Verification items for the finished model (mm, model axes). A direction names the side the tool comes from. Coordinates: 2 decimals unless noted, no trailing zeros. Order: outer loops, then holes, each group sorted by start corner. A loop starts at its lowest first (then second) coordinate and runs counter-clockwise, first axis right, second up.
Q1. Depth check by flat-ended pin: P1, Ø2, axis at x = 69.5, y = -1.5, coming from the +Z side; P2, Ø2, axis at y = 2.5, z = 13.5, coming from the -X side; P3, Ø3, axis at x = 0, y = 0, coming from the -Z side; P4, Ø1, axis at y = 1.5, z = 9.5, coming from the -X side. Enter the tip coordinate at first touch or a pass-through.
Q2. Cross-section at C-C, the plane z = 12.5. Record the boundary of the cut face in (x, y), and give its area (3 significant figures).
Q3. Cross-section at D-D, the plane x = 48.5. Record the boundary of the cut face in (y, z), and give its area (3 significant figures).
Q4. Thickness scan on line 1 (Y direction, x = 135, z = 12.5); line 2 (Y direction, x = 0, z = 2.25); line 3 (X direction, y = -0.25, z = 8.25). Record the ranges inside material, lowest first.
Q5. Cross-section at B-B, the plane x = 19. Record the boundary of the cut face in (y, z).
Q6. Set-up check for faces 4 (the cylindrical face through (28, 0, 4)), 5 (the flat face through (69, 0, 0)): record each of +Z, -Z, +X, -X, +Y, -Y from which the full face is reachable in a straight line by a thin tool's end or side.
Q7. Cross-section at A-A, the plane y = 0. Record the boundary of the cut face in (x, z), and give its area (3 significant figures).
Q8. Draft check along Y on faces 1 (the flat face through (135, -2, 18)), 2 (the flat face through (68, -4, 2)), 3 (the flat face through (13, 0, 3)). Enter one of: pulls with the +Y half, pulls with the -Y half, needs draft (parallel to the pull), parting line crosses it, or undercut.
from build123d import *
from build123d.topology import SkipClean

# Parameters (mm, degrees)
SKETCH2_R           = 2.5
SKETCH2_R_2         = 1.6
BOSS_EXTRUDE1_DEPTH = 5
SKETCH3_R           = 1.6
BOSS_EXTRUDE2_DEPTH = 13
CUT_EXTRUDE1_DEPTH  = 2


with BuildPart() as part:
    # Sketch2 → Boss-Extrude1 (new body)
    with BuildSketch(Plane.XY):
        with BuildLine():
            Line((0, 4), (135, 4))
            ThreePointArc((135, 4), (139, 0), (135, -4))
            Line((135, -4), (0, -4))
            ThreePointArc((0, -4), (-4, 0), (0, 4))
        make_face()
        Circle(SKETCH2_R, mode=Mode.SUBTRACT)
        with Locations((135, 0)):
            Circle(SKETCH2_R_2, mode=Mode.SUBTRACT)
    extrude(amount=BOSS_EXTRUDE1_DEPTH)

    # Sketch3 → Boss-Extrude2 (add)
    with SkipClean():  # the faces are left unmerged after this step: merging them gives an invalid solid
        with BuildSketch(Plane.XY.offset(5)):
            with BuildLine():
                ThreePointArc((135, 4), (131, 0), (135, -4))
                ThreePointArc((135, -4), (139, 0), (135, 4))
            make_face()
            with Locations((135, 0)):
                Circle(SKETCH3_R, mode=Mode.SUBTRACT)
        extrude(amount=BOSS_EXTRUDE2_DEPTH)
    add(part.part.scale(1), mode=Mode.REPLACE)  # the faces are merged on a copy

    # Sketch4 → Cut-Extrude1 (cut)
    with BuildSketch(Plane.XY.offset(5)):
        with BuildLine():
            Line((0, 3), (25, 3))
            ThreePointArc((25, 3), (28, 0), (25, -3))
            Line((25, -3), (0, -3))
            ThreePointArc((0, -3), (-3, 0), (0, 3))
        make_face()
    extrude(amount=-CUT_EXTRUDE1_DEPTH, mode=Mode.SUBTRACT)


solid = part.part
Check values:
1. P1: stops at z = 5
1. P2: stops at x = 131.29
1. P3: passes through
1. P4: stops at x = 131.13
2. outline: circle Ø8 at (135, 0); hole circle Ø3.2 at (135, 0)
2. area: 42.2 mm2
3. outline: (-4, 0) - (4, 0) - (4, 5) - (-4, 5) - close
3. area: 40.0 mm2
4. line 1: y = -4 to -1.6, 1.6 to 4
4. line 2: y = -4 to -2.5, 2.5 to 4
4. line 3: x = 131.01 to 133.42, 136.58 to 138.99
5. outline: (-4, 0) - (4, 0) - (4, 5) - (3, 5) - (3, 3) - (-3, 3) - (-3, 5) - (-4, 5) - close
6. face 4: +Z
6. face 5: -Z, +X, -X, +Y, -Y
7. outline: (-4, 0) - (-2.5, 0) - (-2.5, 3) - (-3, 3) - (-3, 5) - (-4, 5) - close; (2.5, 0) - (133.4, 0) - (133.4, 18) - (131, 18) - (131, 5) - (28, 5) - (28, 3) - (2.5, 3) - close; (136.6, 0) - (139, 0) - (139, 18) - (136.6, 18) - close
7. area: 684 mm2
8. face 1: needs draft
8. face 2: pulls with the -Y half
8. face 3: undercut
